CAD build for the part. Positions are in the model's coordinates, mm. Face numbers are marked on the shaded views. Give positions to 0.01 mm unless a question says otherwise; leave off trailing zeros. Loops run counter-clockwise (first coordinate to the right, second up) from the corner with the lowest first, then second, coordinate; pieces in that order, holes last. Notation, with made-up numbers: (62.5, -40) - (103.5, -40) arc R8 cw to (103.5, -33) - close; hole circle Ø7 at (-11, 37.25). An arc over 180 degrees is marked (long way). Return JSON: item names as keys, results as strings.
from build123d import *

# Parameters (mm, degrees)
SKETCH_1_R          = 0.65
SKETCH_1_R_2        = 1.5
EXTRUDE_1_DEPTH     = 2.3
SKETCH_2_R          = 4.4
EXTRUDE_2_DEPTH     = 3.2
SKETCH_3_R          = 4.4
SKETCH_3_R_2        = 3.4
SKETCH_3_R_3        = 2.75
SKETCH_3_R_4        = 1.5
CUT_EXTRUDE_1_DEPTH = 1
SKETCH1_W           = 12.345584807
SKETCH1_H           = 16.477608666
CUT_EXTRUDE2_DEPTH  = 10


with BuildPart() as part:
    # Эскиз1 → Бобышка-Вытянуть1 (new body)
    with BuildSketch(Plane.XY):
        with BuildLine():
            Line((-3.968626967, 4.5), (-16.888114198, 2.469689731))
            ThreePointArc((-16.888114198, 2.469689731), (-19, 0), (-16.888114198, -2.469689731))
            Line((-16.888114198, -2.469689731), (-3.968626967, -4.5))
            ThreePointArc((-3.968626967, -4.5), (0, -6), (3.968626967, -4.5))
            Line((3.968626967, -4.5), (16.888114198, -2.469689731))
            ThreePointArc((16.888114198, -2.469689731), (19, 0), (16.888114198, 2.469689731))
            Line((16.888114198, 2.469689731), (3.968626967, 4.5))
            ThreePointArc((3.968626967, 4.5), (0, 6), (-3.968626967, 4.5))
        make_face()
        with Locations((-16.5, 0)):
            Circle(SKETCH_1_R, mode=Mode.SUBTRACT)
        with Locations((-13.5, 0)):
            Circle(SKETCH_1_R, mode=Mode.SUBTRACT)
        with Locations((-10.5, 0)):
            Circle(SKETCH_1_R, mode=Mode.SUBTRACT)
        with Locations((-7.5, 0)):
            Circle(SKETCH_1_R, mode=Mode.SUBTRACT)
        with Locations(Location((16.5, 0, 0), (0, 0, 180))):
            Circle(SKETCH_1_R, mode=Mode.SUBTRACT)
        with Locations(Location((7.5, 0, 0), (0, 0, 180))):
            Circle(SKETCH_1_R, mode=Mode.SUBTRACT)
        with Locations(Location((10.5, 0, 0), (0, 0, 180))):
            Circle(SKETCH_1_R, mode=Mode.SUBTRACT)
        with Locations(Location((13.5, 0, 0), (0, 0, 180))):
            Circle(SKETCH_1_R, mode=Mode.SUBTRACT)
        Circle(SKETCH_1_R_2, mode=Mode.SUBTRACT)
    extrude(amount=EXTRUDE_1_DEPTH)

    # Эскиз2 → Бобышка-Вытянуть2 (add)
    with BuildSketch(Plane.XY.offset(2.3)):
        with Locations(Location((0, 0, 0), (0, 0, 180))):
            Circle(SKETCH_2_R)
        Polygon((0.333439775, 2.639447604), (0, 3.05), (-0.333439775, 2.639447604), (-0.758504156, 2.954178641), (-0.979368078, 2.473601404), (-1.469348706, 2.672735374), (-1.563759083, 2.15232973), (-2.087868673, 2.223354314), (-2.049893354, 1.695819264), (-2.575200173, 1.634271725), (-2.407225286, 1.132754236), (-2.900722375, 0.942501833), (-2.6133024, 0.498514094), (-3.043981522, 0.191511085), (-2.655176114, -0.167049522), (-2.995976115, -0.571513009), (-2.530215347, -0.822116802), (-2.75972251, -1.298626839), (-2.246271844, -1.42552746), (-2.35006539, -1.944143169), (-1.821186821, -1.939366985), (-1.792745019, -2.467501833), (-1.281669931, -2.33134895), (-1.122779886, -2.835818282), (-0.661621006, -2.576843686), (-0.382266362, -3.025949839), (0, -2.660425857), (0.382266362, -3.025949839), (0.661621006, -2.576843686), (1.122779886, -2.835818282), (1.281669931, -2.33134895), (1.792745019, -2.467501833), (1.821186821, -1.939366985), (2.35006539, -1.944143169), (2.246271844, -1.42552746), (2.75972251, -1.298626839), (2.530215347, -0.822116802), (2.995976115, -0.571513009), (2.655176114, -0.167049522), (3.043981522, 0.191511085), (2.6133024, 0.498514094), (2.900722375, 0.942501833), (2.407225286, 1.132754236), (2.575200173, 1.634271725), (2.049893354, 1.695819264), (2.087868673, 2.223354314), (1.563759083, 2.15232973), (1.469348706, 2.672735374), (0.979368078, 2.473601404), (0.758504156, 2.954178641), align=None, mode=Mode.SUBTRACT)
    extrude(amount=EXTRUDE_2_DEPTH)

    # Эскиз3 → Вырез-Вытянуть1 (cut)
    # profile 1 of 2: a face of its own
    with BuildSketch(Plane(origin=(0, 0, 0), x_dir=(-1, 0, 0), z_dir=(0, 0, -1))):
        Circle(SKETCH_3_R)
        Circle(SKETCH_3_R_2, mode=Mode.SUBTRACT)
    # profile 2 of 2: a face of its own
    with BuildSketch(Plane(origin=(0, 0, 0), x_dir=(-1, 0, 0), z_dir=(0, 0, -1))):
        Circle(SKETCH_3_R_3)
        Circle(SKETCH_3_R_4, mode=Mode.SUBTRACT)
    extrude(amount=-CUT_EXTRUDE_1_DEPTH, mode=Mode.SUBTRACT)

    # Sketch1 → Cut-Extrude2 (cut)
    with BuildSketch(Plane(origin=(0, 0, 0), x_dir=(-1, 0, 0), z_dir=(0, 0, -1))):
        with Locations((16.022792404, -0.737803373)):
            Rectangle(SKETCH1_W, SKETCH1_H)
    extrude(amount=-CUT_EXTRUDE2_DEPTH, mode=Mode.SUBTRACT)


solid = part.part
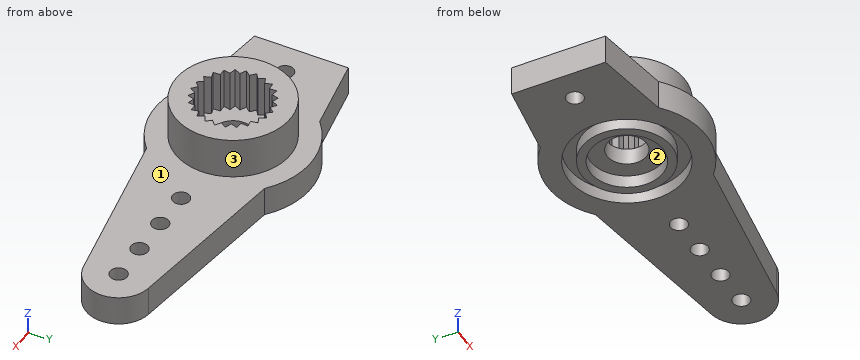
1. Cut at B-B, the plane x = 7.5. Write the cut outline in (y, z).
Values follow:
{"outline": "(-3.95, 0) - (-0.65, 0) - (-0.65, 2.3) - (-3.95, 2.3) - close; (0.65, 0) - (3.95, 0) - (3.95, 2.3) - (0.65, 2.3) - close"}
2. Cut at C-C, the plane x = 10.5. Write the cut outline in (y, z).
Values follow:
{"outline": "(-3.47, 0) - (-0.65, 0) - (-0.65, 2.3) - (-3.47, 2.3) - close; (0.65, 0) - (3.47, 0) - (3.47, 2.3) - (0.65, 2.3) - close"}
3. Drill centre lines: probe 1 along X at (y, z) = (2.75, 4.9); probe 2 along Y at (x, z) = (0, 0.45); probe 3 along Y at (x, z) = (-3.5, 0.45). Where is each one in solid material? Low to high.
Values follow:
{"probe 1": "x = -3.43 to -0.85, -0.48 to -0.24, 0.24 to 0.48, 0.85 to 3.43", "probe 2": "y = -6 to -4.4, -3.4 to -2.75, 2.75 to 3.4, 4.4 to 6", "probe 3": "y = -4.87 to -2.67, 2.67 to 4.87"}
4. Cut at D-D, the plane x = -6. Write the cut outline in (y, z), plus the area to 3 significant figures.
Values follow:
{"outline": "(-4.18, 0) - (4.18, 0) - (4.18, 2.3) - (-4.18, 2.3) - close", "area": "19.2 mm²"}
5. Pull direction Y, two halves, no side cores. Call the marked faces 1, 2 and 3: +Y half, -Y half, draft (parallel to the pull), parting line (faces both ways), or undercut.
Values follow:
{"face 1": "draft", "face 2": "undercut", "face 3": "parting line"}
6. Cut at A-A, the plane z = 2. Write the cut outline in (x, y).
Values follow:
{"outline": "(-9.85, -3.58) - (-3.97, -4.5) arc R6 ccw to (3.97, -4.5) - (16.89, -2.47) arc R2.5 ccw to (16.89, 2.47) - (3.97, 4.5) arc R6 ccw to (-3.97, 4.5) - (-9.85, 3.58) - close; hole circle Ø1.3 at (-7.5, 0); hole circle Ø3 at (0, 0); hole circle Ø1.3 at (7.5, 0); hole circle Ø1.3 at (10.5, 0); hole circle Ø1.3 at (13.5, 0); hole circle Ø1.3 at (16.5, 0)"}
7. Drop flat-ended pins along their axis: P1, Ø1.2, axis at x = 10.5, y = 0, coming from the +Z side; P2, Ø3, axis at x = 10.5, y = 2.5, coming from the +Z side; P3, Ø2, axis at x = 1, z = 3.5, coming from the +Y side; P4, Ø1.5, axis at y = 4, z = 3.5, coming from the -X side. Give the stop position or say it passes through.
Values follow:
{"P1": "passes through", "P2": "stops at z = 2.3", "P3": "stops at y = 4.4", "P4": "stops at x = -2.97"}
